from build123d import *

# Parameters (mm, degrees)
CROQUIS1_R              = 3.75
CROQUIS1_R_2            = 1.65
SALIENTE_EXTRUIR1_DEPTH = 2
SALIENTE_EXTRUIR2_DEPTH = 2
CROQUIS5_R              = 1.65
CROQUIS5_R_2            = 1.7
CORTAR_EXTRUIR2_DEPTH   = 10
REDONDEO3_R             = 1
REDONDEO4_R             = 1
REDONDEO5_R             = 1
REDONDEO6_R             = 1
REDONDEO7_R             = 1
REDONDEO8_R             = 1
REDONDEO12_R            = 2


with BuildPart() as part:
    # Croquis1 → Saliente-Extruir1 (new body)
    with BuildSketch(Plane.XY):
        with BuildLine():
            Line((0, 0), (0, 25))
            Line((0, 25), (14.5, 25))
            ThreePointArc((14.5, 25), (27, 12.5), (14.5, 0))
            Line((14.5, 0), (0, 0))
        make_face()
        with Locations((14.5, 12.5)):
            Circle(CROQUIS1_R, mode=Mode.SUBTRACT)
        with Locations((14.5, 21)):
            Circle(CROQUIS1_R_2, mode=Mode.SUBTRACT)
        with Locations((23, 12.5)):
            Circle(CROQUIS1_R_2, mode=Mode.SUBTRACT)
        with Locations((14.5, 4)):
            Circle(CROQUIS1_R_2, mode=Mode.SUBTRACT)
        with Locations((6, 12.5)):
            Circle(CROQUIS1_R_2, mode=Mode.SUBTRACT)
    extrude(amount=SALIENTE_EXTRUIR1_DEPTH)

    # Croquis4 → Saliente-Extruir2 (add)
    with BuildSketch(Plane.ZY):
        with BuildLine():
            Line((2, 0), (-46.922808665, 0))
            ThreePointArc((-46.922808665, 0), (-48.82286243, 0.503124666), (-50, 2.077191335))
            Line((-50, 2.077191335), (-50, 22.665501207))
            ThreePointArc((-50, 22.665501207), (-49.183232344, 24.133251816), (-47.715481735, 24.950019472))
            Line((-47.715481735, 24.950019472), (2, 24.950019472))
            Line((2, 24.950019472), (2, 0))
        make_face()
    extrude(amount=-SALIENTE_EXTRUIR2_DEPTH)

    # Croquis5 → Cortar-Extruir2 (cut)
    with BuildSketch(Plane(origin=(2, 0, 0), x_dir=(0, 0, -1), z_dir=(1, 0, 0))):
        with Locations((42.5, 12.371346271)):
            Circle(CROQUIS5_R)
        with Locations((36.15, 12.371346271)):
            Circle(CROQUIS5_R)
        with Locations((29.8, 12.371346271)):
            Circle(CROQUIS5_R)
        with Locations((23.45, 12.371346271)):
            Circle(CROQUIS5_R)
        with Locations((17.1, 12.371346271)):
            Circle(CROQUIS5_R)
        with Locations((10.75, 12.371346271)):
            Circle(CROQUIS5_R)
        with Locations((4.4, 12.371346271)):
            Circle(CROQUIS5_R)
        with Locations((7.5, 23.35)):
            Circle(CROQUIS5_R_2)
        with Locations((13.85, 23.35)):
            Circle(CROQUIS5_R_2)
        with Locations((20.2, 23.35)):
            Circle(CROQUIS5_R_2)
        with Locations((26.55, 23.35)):
            Circle(CROQUIS5_R_2)
        with Locations((32.9, 23.35)):
            Circle(CROQUIS5_R_2)
        with Locations((39.25, 23.35)):
            Circle(CROQUIS5_R_2)
        with Locations((39.25, 1.392692542)):
            Circle(CROQUIS5_R_2)
        with Locations((32.9, 1.392692542)):
            Circle(CROQUIS5_R_2)
        with Locations((26.55, 1.392692542)):
            Circle(CROQUIS5_R_2)
        with Locations((20.2, 1.392692542)):
            Circle(CROQUIS5_R_2)
        with Locations((13.85, 1.392692542)):
            Circle(CROQUIS5_R_2)
        with Locations((7.5, 1.392692542)):
            Circle(CROQUIS5_R_2)
    extrude(amount=-CORTAR_EXTRUIR2_DEPTH, mode=Mode.SUBTRACT)

    # Redondeo3
    redondeo3_edges = [part.edges().sort_by_distance(p)[0] for p in [
        (1, 24.950019472, -8.074402028),
        (1, 24.950019472, -13.275597972),
    ]]
    fillet(redondeo3_edges, radius=REDONDEO3_R)

    # Redondeo4
    redondeo4_edges = [part.edges().sort_by_distance(p)[0] for p in [
        (1, 24.950019472, -19.625597972),
        (1, 24.950019472, -20.774402028),
        (1, 24.950019472, -25.975597972),
        (1, 24.950019472, -14.424402028),
    ]]
    fillet(redondeo4_edges, radius=REDONDEO4_R)

    # Redondeo5
    redondeo5_edges = [part.edges().sort_by_distance(p)[0] for p in [
        (1, 24.950019472, -32.325597972),
        (1, 24.950019472, -33.474402028),
        (1, 24.950019472, -38.675597972),
        (1, 24.950019472, -39.824402028),
        (1, 24.950019472, -27.124402028),
    ]]
    fillet(redondeo5_edges, radius=REDONDEO5_R)

    # Redondeo6
    redondeo6_edges = [part.edges().sort_by_distance(p)[0] for p in [
        (1, 24.950019472, -6.925597972),
    ]]
    fillet(redondeo6_edges, radius=REDONDEO6_R)

    # Redondeo7
    redondeo7_edges = [part.edges().sort_by_distance(p)[0] for p in [
        (1, 0, -31.925111553),
        (1, 0, -25.575111553),
        (1, 0, -27.524888447),
        (1, 0, -19.225111553),
        (1, 0, -21.174888447),
        (1, 0, -12.875111553),
        (1, 0, -14.824888447),
        (1, 0, -6.525111553),
        (1, 0, -8.474888447),
    ]]
    fillet(redondeo7_edges, radius=REDONDEO7_R)

    # Redondeo8
    redondeo8_edges = [part.edges().sort_by_distance(p)[0] for p in [
        (1, 0, -38.275111553),
        (1, 0, -40.224888447),
        (1, 0, -33.874888447),
    ]]
    fillet(redondeo8_edges, radius=REDONDEO8_R)

    # Redondeo12
    redondeo12_edges = [part.edges().sort_by_distance(p)[0] for p in [
        (0, 12.5, 2),
    ]]
    fillet(redondeo12_edges, radius=REDONDEO12_R)


solid = part.part
Geometry check sheet. Reference: the model listing, model coordinates, mm. A direction names the side the tool comes from. Round coordinates to 2 decimals unless told otherwise and drop trailing zeros. Order: outer loops, then holes, each group sorted by start corner. A loop starts at its lowest first (then second) coordinate and runs counter-clockwise, first axis right, second up. Notation, with made-up numbers: M -29.75,18 L -23.75,18 A29 ccw -23.75,42 Z; hole C 88,89 d7. An arc over 180 degrees is marked long. Write each question's results on one line, items separated by ' | '. Start each with the question number.
1. Draft check along Z on faces 1 (the face through (0.986, 24.116, -49.2)), 2 (the face through (1.01, 0.34, -37.33)), 3 (the face through (11.736, 15.034, 0.986)). Enter one of: pulls with the +Z half, pulls with the -Z half, needs draft (parallel to the pull), parting line crosses it, or undercut.
2. Cross-section at B-B on x = 13.75. Record the boundary of the cut face in (y, z).
3. Material ranges on L1, parallel to Y at x = 14.5, z = 0.6; L2, parallel to Y at x = 1.1, z = -4.4; L3, parallel to Z at x = 19.5, y = 5, recorded low to high. Write a range as from..to.
4. Cross-section at D-D on y = 18.25. Record the boundary of the cut face in (x, z), plus the area to 3 significant figures.
5. Go/stop test with flat-tipped pins: P1, Ø1.5, axis at x = 13, y = 15.5, coming from the -Z side; P2, Ø3, axis at y = 12.37, z = -42.5, coming from the -X side; P3, Ø0.5, axis at x = 1, z = -23.5, coming from the +Y side; P4, Ø5.5, axis at y = 1.39, z = -32.9, coming from the +X side. Record where each tip stops, or that it passes through.
6. Cross-section at A-A on z = -42.5. Record the boundary of the cut face in (x, y).
7. Set-up check for faces 4 (the face through (1.014, 3.092, -7.541)), 5 (the face through (1, 24.95, -17)): record each of +Z, -Z, +X, -X, +Y, -Y from which the full face is reachable in a straight line by a thin tool's end or side.
8. Cross-section at C-C on y = 15.5. Record the boundary of the cut face in (x, z), plus the area to 3 significant figures.
Resolved:
1) face 1: pulls with the -Z half | face 2: undercut | face 3: needs draft
2) outline: M 0,0 L 2.53,0 L 2.53,2 L 0,2 Z; M 5.47,0 L 8.83,0 L 8.83,2 L 5.47,2 Z; M 16.17,0 L 19.53,0 L 19.53,2 L 16.17,2 Z; M 22.47,0 L 25,0 L 25,2 L 22.47,2 Z
3) L1: 0..2.35, 5.65..8.75, 16.25..19.35, 22.65..25 | L2: 0..10.72, 14.02..24.95 | L3: 0..2
4) outline: M 0,-50 L 2,-50 L 2,0 L 25.6,0 L 25.6,2 L 2,2 A2 ccw 0,0 Z | area: 150 mm2
5) P1: z = 0 | P2: through | P3: y = 24.95 | P4: x = 2
6) outline: M 0,0 L 2,0 L 2,10.72 L 0,10.72 Z; M 0,14.02 L 2,14.02 L 2,24.95 L 0,24.95 Z
7) face 4: +X, -X | face 5: -Z, +X, -X, +Y
8) outline: M 0,-50 L 2,-50 L 2,0 L 12.25,0 L 12.25,2 L 2,2 A2 ccw 0,0 Z; M 16.75,0 L 26.63,0 L 26.63,2 L 16.75,2 Z | area: 143 mm2
